Geometry check sheet. Reference: the model listing, model coordinates, mm. Face numbers are marked on the shaded views. Coordinates: 2 decimals unless noted, no trailing zeros. Loops run counter-clockwise (first coordinate to the right, second up) from the corner with the lowest first, then second, coordinate; pieces in that order, holes last. Notation, with made-up numbers: (-0.75, -33.75) -> (39.25, -33.75) arc R27 cw to (39.25, -0.75) -> close; hole circle Ø11 at (-5.5, 15.5). An arc over 180 degrees is marked (long way). Answer as a JSON object with one key per item and string values.
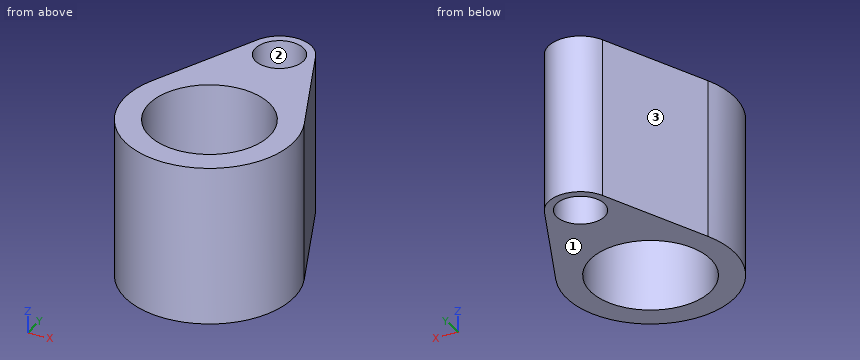
from build123d import *

# Parameters (mm, degrees)
SKETCH1_R           = 75
BOSS_EXTRUDE1_DEPTH = 100
SKETCH3_R           = 30
CUT_EXTRUDE2_DEPTH  = 349.20970693


with BuildPart() as part:
    # Sketch1 → Boss-Extrude1 (new, symmetric)
    with BuildSketch(Plane.XY):
        with BuildLine():
            Line((-95.945006832, -117.34375), (-36.550478793, 16.25))
            ThreePointArc((-36.550478793, 16.25), (0, 40), (36.550478793, 16.25))
            Line((36.550478793, 16.25), (95.945006832, -117.34375))
            ThreePointArc((95.945006832, -117.34375), (0, -265), (-95.945006832, -117.34375))
        make_face()
        with Locations((0, -160)):
            Circle(SKETCH1_R, mode=Mode.SUBTRACT)
    extrude(amount=BOSS_EXTRUDE1_DEPTH, both=True)

    # Sketch3 → Cut-Extrude2 (cut, through all)
    with BuildSketch(Plane.XY.offset(100)):
        Circle(SKETCH3_R)
    extrude(amount=-CUT_EXTRUDE2_DEPTH, mode=Mode.SUBTRACT)


solid = part.part
1. Mould release check, pull along Y, two halves, no side actions. Record for the marked faces 1, 2 and 3: released by +Y, released by -Y, zero draft, split by the parting line, or undercut.
Evaluation:
{"face 1": "zero draft", "face 2": "undercut", "face 3": "released by +Y"}
2. Section check B-B, the plane z = 48. Record the boundary of the cut face in (x, y) (3 decimals).
Evaluation:
{"outline": "(-95.945, -117.344) arc R105 ccw (long way) to (95.945, -117.344) -> (36.55, 16.25) arc R40 ccw to (-36.55, 16.25) -> close; hole circle Ø150 at (0, -160); hole circle Ø60 at (0, 0)"}
3. Section check A-A, the plane y = -160. Record the boundary of the cut face in (x, z).
Evaluation:
{"outline": "(-105, -100) -> (-75, -100) -> (-75, 100) -> (-105, 100) -> close; (75, -100) -> (105, -100) -> (105, 100) -> (75, 100) -> close"}
4. Section check C-C, the plane x = 0. Record the boundary of the cut face in (y, z).
Evaluation:
{"outline": "(-265, -100) -> (-235, -100) -> (-235, 100) -> (-265, 100) -> close; (-85, -100) -> (-30, -100) -> (-30, 100) -> (-85, 100) -> close; (30, -100) -> (40, -100) -> (40, 100) -> (30, 100) -> close"}
5. Thickness scan on probe 1 along Y at (x, z) = (0, 45); probe 2 along Y at (x, z) = (-16, -72.5); probe 3 along X at (y, z) = (-158, -14). Record the ranges inside material, lowest first. Write a range as from..to.
Evaluation:
{"probe 1": "y = -265..-235, -85..-30, 30..40", "probe 2": "y = -263.77..-233.27, -86.73..-25.38, 25.38..36.66", "probe 3": "x = -104.98..-74.97, 74.97..104.98"}
6. Section check D-D, the plane y = 0. Record the boundary of the cut face in (x, z), then the cut area to 3 significant figures.
Evaluation:
{"outline": "(-43.78, -100) -> (-30, -100) -> (-30, 100) -> (-43.78, 100) -> close; (30, -100) -> (43.78, -100) -> (43.78, 100) -> (30, 100) -> close", "area": "5,510 mm^2"}
7. Depth check by flat-ended pin: P1, Ø2, axis at x = 35, z = -25, coming from the -Y side; P2, Ø1, axis at y = -64.5, z = 49, coming from the +X side; P3, Ø1, axis at x = -70.5, z = -12.5, coming from the -Y side. Enter the tip coordinate at first touch or a pass-through.
Evaluation:
{"P1": "stops at y = -259.34", "P2": "stops at x = 72.67", "P3": "stops at y = -238.26"}
